Input: part model. Units: mm. Frame: model coordinates. Face numbers are marked on the shaded views. A direction names the side the tool comes from. Give positions to 0.01 mm unless a question says otherwise; leave off trailing zeros. Loops run counter-clockwise (first coordinate to the right, second up) from the corner with the lowest first, then second, coordinate; pieces in that order, holes last. Notation, with made-up numbers: (42.5, 29.5) -> (61.5, 29.5) arc R27 cw to (61.5, 58.5) -> close; hole circle Ø9 at (-30.75, 66.5). An arc over 180 degrees is marked (long way). One line per question, with ' | ' between items.
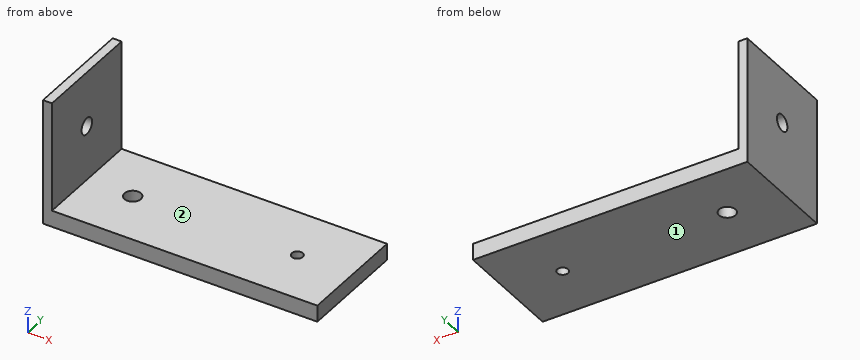
from build123d import *

# Parameters (mm, degrees)
F0_W     = 50
F0_H     = 20
F0_R     = 1.5
F0_R_2   = 1
F1_DEPTH = 3
F2_W     = 1.635674
F2_H     = 20
F3_DEPTH = 20
F5_D     = 3


with BuildPart() as f1:
    # F0 (on Top) → F1 (new body)
    with BuildSketch(Plane.XY):
        Rectangle(F0_W, F0_H)
        with Locations((-15, 0)):
            Circle(F0_R, mode=Mode.SUBTRACT)
        with Locations((15, 0)):
            Circle(F0_R_2, mode=Mode.SUBTRACT)
    extrude(amount=F1_DEPTH)

    # F2 (on face) → F3 (join)
    with BuildSketch(Plane.XY.offset(3)):
        with Locations((-24.182163, 0)):
            Rectangle(F2_W, F2_H)
    extrude(amount=F3_DEPTH)

    # F5 (through all)
    with Locations(Plane.YZ.offset(-23.364326)):
        with Locations((0, 13)):
            Hole(F5_D / 2)


solid = f1.part
1. Section query B-B (y = 0). Output: boundary loops of the cut face in (x, z).
Determined:
outline: (-25, 0) -> (-16.5, 0) -> (-16.5, 3) -> (-23.36, 3) -> (-23.36, 11.5) -> (-25, 11.5) -> close; (-25, 14.5) -> (-23.36, 14.5) -> (-23.36, 23) -> (-25, 23) -> close; (-13.5, 0) -> (14, 0) -> (14, 3) -> (-13.5, 3) -> close; (16, 0) -> (25, 0) -> (25, 3) -> (16, 3) -> close
2. Reachability of the marked faces 1 and 2 from +Z, -Z, +X, -X, +Y, -Y: full face, straight path, thin tool, end or side. Return the list, or none.
Determined:
face 1: -Z, +X, -X, +Y, -Y | face 2: +Z, +X, +Y, -Y
3. Section query C-C (z = 13). Output: boundary loops of the cut face in (x, y).
Determined:
outline: (-25, -10) -> (-23.36, -10) -> (-23.36, -1.5) -> (-25, -1.5) -> close; (-25, 1.5) -> (-23.36, 1.5) -> (-23.36, 10) -> (-25, 10) -> close
4. Pin query (flat end, axial travel): P1, Ø1, axis at x = 7.5, y = 5.5, coming from the -Z side; P2, Ø8, axis at y = -3.5, z = 13, coming from the +X side; P3, Ø2.5, axis at y = 0, z = 13, coming from the -X side. Return the tip coordinate at first contact, or that it passes through.
Determined:
P1: stops at z = 0 | P2: stops at x = -23.36 | P3: passes through
5. Section query D-D (y = -8.5). Output: boundary loops of the cut face in (x, z), then the cut area to 3 significant figures.
Determined:
outline: (-25, 0) -> (25, 0) -> (25, 3) -> (-23.36, 3) -> (-23.36, 23) -> (-25, 23) -> close | area: 183 mm2
6. Section query A-A (x = 15). Output: boundary loops of the cut face in (y, z).
Determined:
outline: (-10, 0) -> (-1, 0) -> (-1, 3) -> (-10, 3) -> close; (1, 0) -> (10, 0) -> (10, 3) -> (1, 3) -> close
7. Ray query, line 1 along Z through (x, y) = (-24.2, 0); line 2 along Y through (x, z) = (-15, 2.35); line 3 along Y through (x, z) = (15, 0.8). Return the intervals inside material, ascending. Write a range as from..to.
Determined:
line 1: z = 0..11.5, 14.5..23 | line 2: y = -10..-1.5, 1.5..10 | line 3: y = -10..-1, 1..10
